CAD build for the part. Positions are in the model's coordinates, mm. Face numbers are marked on the shaded views. A direction names the side the tool comes from. Give positions to 0.01 mm unless a question says otherwise; leave off trailing zeros. Order: outer loops, then holes, each group sorted by start corner. A loop starts at its lowest first (then second) coordinate and runs counter-clockwise, first axis right, second up. Notation, with made-up numbers: M 4.25,-23.5 L 51.25,-23.5 A12 ccw 51.25,-19.5 Z; hole C 79.5,-19.5 d11. An arc over 180 degrees is marked long. Put each result on its own line as item: value. Start each with the question number.
1) Cut at D-D (z = 5.25). Write the cut outline in (x, y).
2) Cut at A-A (y = 47). Write the cut outline in (x, z).
3) Tool access for the marked faces 1, 2 and 3: list every direction of +Z, -Z, +X, -X, +Y, -Y with a clear straight run to the whole face (end or side of a thin tool).
4) Drill centre lines: line 1 (X direction, y = 47, z = 20.4); line 2 (Z direction, x = 5.5, y = 35.5); line 3 (Z direction, x = 9, y = 6.5). Where is each one in solid material? Low to high. Write a range as [from, to].
5) Cut at C-C (x = 4.5). Write the cut outline in (y, z).
6) Pin check, flat tips, straight feed: pin 1 (8.5 mm diameter, centred on x = 6, z = 11.5, fed in from -Y); pin 2 (15 mm diameter, centred on x = -1, y = 41.5, fed in from -Z); pin 3 (12 mm diameter, centred on x = -11, y = 16.5, fed in from +Z). Stop position of each tip, or through.
7) Cut at B-B (x = -7.5). Write the cut outline in (y, z).
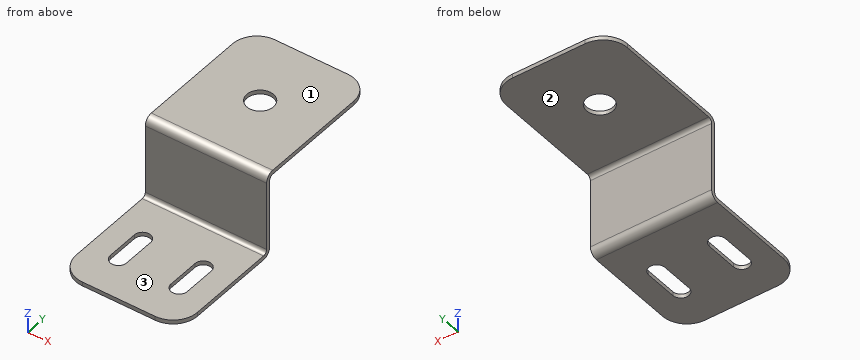
Autodesk Inventor part; units mm, degrees
ref_plane "YZ Plane" through (0, 0, 0) normal (1, 0, 0) x (0, 1, 0)
ref_plane "XZ Plane" through (0, 0, 0) normal (0, 1, 0) x (-1, 0, 0)
ref_plane "XY Plane" through (0, 0, 0) normal (0, 0, 1) x (1, 0, 0)
sketch "Skizze1" plane through (0, 0, 0) normal (0, 0, 1) x (1, 0, 0)
  line L0 (-15, 30) -> (15, 30)
  line L1 (15, 30) -> (15, 0)
  line L2 (15, 0) -> (-15, 0)
  line L3 (-15, 0) -> (-15, 30)
  line L4 (-15, 30) -> (15, 0) construction
  line L5 (15, 30) -> (-15, 0) construction
  point P0 (0, 0)
  point P1 (0, 15)
  dimension "d0" = 30
  dimension "d1" = 30
extrude "Grobblech1" add sketch "Skizze1" along normal blind 1
sketch "Skizze2" plane through (-15, 29, 0) normal (0, 1, 0) x (-1, 0, 0)
  line L0 (-30, 0) -> (0, 0)
  line L1 (0, 0) -> (0, 21)
  line L2 (0, 21) -> (-30, 21)
  line L3 (-30, 21) -> (-30, 0)
edge flange "Lasche1" height 20 angle 90 thickness 1 bend radius 1 thickness toward (0, 1, 0) relief tear relief width 1 relief depth 0.5 edges at (0, 30, 1) wall of the first edge with corners at (15, 29, 0) (-15, 29, 0) (-15, 29, 21) (15, 29, 21)
bend "Biegung1"
corner "Ecke1"
sketch "Skizze3" plane through (15, 29, 20) normal (0, 0, 1) x (1, 0, 0)
  line L0 (-30, 0) -> (0, 0)
  line L1 (0, 0) -> (0, 35)
  line L2 (0, 35) -> (-30, 35)
  line L3 (-30, 35) -> (-30, 0)
edge flange "Lasche2" height 34 angle 90 thickness 1 bend radius 1 thickness toward (0, 0, 1) relief tear relief width 1 relief depth 0.5 edges at (0, 30, 21) wall of the first edge with corners at (-15, 29, 20) (15, 29, 20) (15, 64, 20) (-15, 64, 20)
bend "Biegung2"
corner "Ecke2"
hole "Bohrung2" at (0, 47, 21) direction (0, 0, -1) diameter 6.6 end through all
sketch "Skizze6" plane through (0, 0, 1) normal (0, 0, 1) x (1, 0, 0)
  line L0 (15, 28) -> (-15, 28)
  line L1 (-15, 0) -> (-15, 28)
  line L2 (7.5, 10) -> (7.5, 18) construction
  line L3 (9.5, 10) -> (9.5, 18)
  line L4 (5.5, 18) -> (5.5, 10)
  arc A0 (5.5, 10) -> (9.5, 10) centre (7.5, 10) ccw
  arc A1 (9.5, 18) -> (5.5, 18) centre (7.5, 18) ccw
  line L5 (0, 28) -> (0, 0) construction
  line L6 (-7.5, 10) -> (-7.5, 18) construction
  line L7 (-9.5, 10) -> (-9.5, 18)
  line L8 (-5.5, 18) -> (-5.5, 10)
  arc A2 (-9.5, 10) -> (-5.5, 10) centre (-7.5, 10) ccw
  arc A3 (-5.5, 18) -> (-9.5, 18) centre (-7.5, 18) ccw
  point P0 (7.5, 14)
  point P1 (-7.5, 14)
  point P2 (0, 14)
  dimension "d47" = 15
  dimension "d48" = 12
  dimension "d50" = 4
extrude "Extrusion2" cut sketch "Skizze6" against normal through all
fillet "Eckenrundung1" radius 6 4 edges at (15, 0, 0.5) (-15, 0, 0.5) (-15, 64, 20.5) (15, 64, 20.5)
equation "\"d45\" = Stärke"
equation "\"d3\" = BreiteBiegungsfreistellung"
equation "\"d4\" = TiefeBiegungsfreistellung"
equation "\"d5\" = MinimalRest"
equation "\"d6\" = Biegeradius"
equation "\"d9\" = Biegeradius"
equation "\"d10\" = GrößeEckenfreistellung"
equation "\"d11\" = Abstandsgröße"
equation "\"d12\" = JacobiRadiusGröße"
equation "\"d13\" = BreiteBiegungsfreistellung"
equation "\"d14\" = TiefeBiegungsfreistellung"
equation "\"d15\" = MinimalRest"
equation "\"d16\" = Biegeradius"
equation "\"d19\" = Biegeradius"
equation "\"d20\" = GrößeEckenfreistellung"
equation "\"d21\" = Abstandsgröße"
equation "\"d22\" = JacobiRadiusGröße"
equation "\"Biegeradius\" = Stärke"
equation "\"BreiteBiegungsfreistellung\" = Stärke"
equation "\"TiefeBiegungsfreistellung\" = 0.5 * Stärke"
equation "\"GrößeEckenfreistellung\" = 4 * Stärke"
equation "\"MinimalRest\" = 2 * Stärke"
equation "\"Übergangsradius\" = Biegeradius"
equation "\"JacobiRadiusGröße\" = Biegeradius"
equation "\"Abstandsgröße\" = Stärke"
equation "\"d2\" = Biegeradius"
properties part number "Tunel_IRBeamHolder"
Solution:
1. outline: M -15,29 L 15,29 L 15,30 L -15,30 Z
2. outline: M -15,20 L -3.3,20 L -3.3,21 L -15,21 Z; M 3.3,20 L 15,20 L 15,21 L 3.3,21 Z
3. face 1: +Z, +X, -X, +Y, -Y
3. face 2: -Z, +X, -X, +Y
3. face 3: +Z, +X, -X, -Y
4. line 1: [-15, -3.3], [3.3, 15]
4. line 2: [20, 21]
4. line 3: [0, 1]
5. outline: M 0,0 L 28,0 A2 ccw 30,2 L 30,19 A1 cw 31,20 L 64,20 L 64,21 L 31,21 A2 ccw 29,19 L 29,2 A1 cw 28,1 L 0,1 Z
6. pin 1: y = 29
6. pin 2: z = 20
6. pin 3: z = 1
7. outline: M 0,0 L 8,0 L 8,1 L 0,1 Z; M 20,0 L 28,0 A2 ccw 30,2 L 30,19 A1 cw 31,20 L 64,20 L 64,21 L 31,21 A2 ccw 29,19 L 29,2 A1 cw 28,1 L 20,1 Z
